The listing builds one solid part. Answer for the finished solid, in the listing's coordinates (mm). A direction names the side the tool comes from. Give positions to 0.01 mm unless a question says otherwise; leave off trailing zeros. Write each loop counter-clockwise with the first axis right and the second up, starting at its lowest first coordinate (ties: lowest second). Pieces come first, ordered by that corner, then holes. Notation, with made-up numbers: M 49,20 L 100,20 A21 ccw 100,55 Z; hole C -10,88.5 d3. An arc over 180 degrees is marked long. Return JSON: item names as keys, results as strings.
Autodesk Inventor part; units mm, degrees
ref_plane "YZ Plane" through (0, 0, 0) normal (1, 0, 0) x (0, 1, 0)
ref_plane "XZ Plane" through (0, 0, 0) normal (0, 1, 0) x (-1, 0, 0)
ref_plane "XY Plane" through (0, 0, 0) normal (0, 0, 1) x (1, 0, 0)
ref_plane "작업 평면1" through (0, 0, 0) normal (0, 0, 1) x (1, 0, 0)
sketch "스케치1" plane through (0, 0, 0) normal (0, 0, 1) x (1, 0, 0)
  circle A0 centre (-7.7782, -7.7782) radius 1.55
  circle A1 centre (7.7782, -7.7782) radius 1.55
  circle A2 centre (7.7782, 7.7782) radius 1.55
  circle A3 centre (-7.7782, 7.7782) radius 1.55
  circle A4 centre (0, 0) radius 5
  circle A5 centre (0, 0) radius 13.9
  circle A6 centre (0, 11) radius 1.55
  circle A7 centre (11, 0) radius 1.55
  circle A8 centre (0, -11) radius 1.55
  circle A9 centre (-11, 0) radius 1.55
  line L0 (13.9, 0) -> (13.9, 13.9)
  line L1 (13.9, 13.9) -> (-13.9, 13.9)
  line L2 (-13.9, 13.9) -> (13.9, 13.9)
  line L3 (13.9, 28.9) -> (-13.9, 28.9)
  line L4 (3.1, 28.9) -> (-3.1, 28.9)
  circle A10 centre (0, 0) radius 5.1
  circle A11 centre (-7.7782, 7.7782) radius 1.35
  circle A12 centre (-11, 0) radius 1.35
  circle A13 centre (-7.7782, -7.7782) radius 1.35
  circle A14 centre (0, -11) radius 1.35
  circle A15 centre (7.7782, -7.7782) radius 1.35
  circle A16 centre (11, 0) radius 1.35
  circle A17 centre (7.7782, 7.7782) radius 1.35
  circle A18 centre (0, 11) radius 1.35
  circle A19 centre (0, 0) radius 13.9
  line L5 (-5.1, 0) -> (-5.1, -12.9306)
  line L6 (5.1, 0) -> (5.1, -12.9306)
  line L7 (6.05, 28.9) -> (-6.05, 28.9)
  line L8 (-6.05, 28.9) -> (-6.05, 22.8)
  line L9 (-6.05, 22.8) -> (6.05, 22.8)
  line L10 (6.05, 22.8) -> (6.05, 28.9)
  line L11 (13.9, 28.9) -> (20.9, 28.9)
  line L12 (20.9, 28.9) -> (20.9, 13.9)
  line L13 (20.9, 13.9) -> (13.9, 13.9)
  line L14 (-13.9, 28.9) -> (-20.9, 28.9)
  line L15 (-20.9, 28.9) -> (-20.9, 13.9)
  line L16 (-20.9, 13.9) -> (-13.9, 13.9)
  line L17 (-20.9, 13.9) -> (-13.9, 0)
  line L18 (13.9, 0) -> (20.9, 13.9)
  circle A20 centre (-10.9, 25.9) radius 1.35
  circle A21 centre (10.9, 25.9) radius 1.35
  point P0 (0, 0)
  point P1 (0, 13.9)
  dimension "d24" = 0.1
  dimension "d25" = 2.7
  dimension "d28" = 360
  dimension "d30" = 12.1
  dimension "d31" = 6.1
  dimension "d39" = 2.7
  dimension "d40" = 2.7
extrude "돌출7" add sketch "스케치1" along normal blind 6 contours A0 | A1 | A2 | A3 | A5 L6 A10 L5 | L17 L16 L1 A5 | L1 L0 A5 | L1 L16 L15 L14 L3 L8 L9 L10 L11 L12 L13 | L0 L13 L18 | A6 | A7 | A9 picked at (-7.5104, -2.4224)
fillet "모깎기3" radius 1 2 edges at (-5.1, -12.9306, 3) (5.1, -12.9306, 3)
sketch "스케치2" plane through (0, 0, 6) normal (0, 0, 1) x (1, 0, 0)
  line L0 (-6.05, 22.8) -> (-6.05, 28.9)
  line L1 (6.05, 22.8) -> (-6.05, 22.8)
  line L2 (6.05, 28.9) -> (6.05, 22.8)
  circle A0 centre (-6.05, 22.8) radius 1
  circle A1 centre (6.05, 22.8) radius 1
  point P0 (0, 0)
  dimension "d47" = 2
  dimension "d48" = 2
extrude "돌출8" cut sketch "스케치2" against normal blind 10
properties part number "leg_between_64" material "PMMA 플라스틱"
Item 1: Find the intervals of material crossed by line 1 (Y direction, x = -8, z = 1.9); line 2 (Y direction, x = -11, z = 3.55); line 3 (X direction, y = 27, z = 5.75), in increasing order.
Geometry results:
{"line 1": "y = -11.37 to -9.11, -6.45 to 6.45, 9.11 to 28.9", "line 2": "y = -8.5 to -1.35, 1.35 to 24.55, 27.25 to 28.9", "line 3": "x = -20.9 to -11.68, -10.12 to -6.05, 6.05 to 10.12, 11.68 to 20.9"}
Item 2: A cutting plane is placed at C-C, the plane z = 4.9. Count the separate pieces of the cut face and the enclosed holes in it, plus the area to 3 significant figures.
Geometry results:
{"separate pieces": "1", "enclosed holes": "9", "area": "1,100 mm2"}
Item 3: A cutting plane is placed at B-B, the plane x = 0. Write down the section's boundary in (y, z), plus the area to 3 significant figures.
Geometry results:
{"outline": "M 5.1,0 L 9.65,0 L 9.65,6 L 5.1,6 Z; M 12.35,0 L 22.8,0 L 22.8,6 L 12.35,6 Z", "area": "90.0 mm2"}
Item 4: A cutting plane is placed at A-A, the plane y = 25.9. Write down the section's boundary in (x, z), plus the area to 3 significant figures.
Geometry results:
{"outline": "M -20.9,0 L -12.25,0 L -12.25,6 L -20.9,6 Z; M -9.55,0 L -6.05,0 L -6.05,6 L -9.55,6 Z; M 6.05,0 L 9.55,0 L 9.55,6 L 6.05,6 Z; M 12.25,0 L 20.9,0 L 20.9,6 L 12.25,6 Z", "area": "146 mm2"}
Item 5: Which of the six approach directions +Z, -Z, +X, -X, +Y, -Y give full straight-line access (tool end or side, diameter ignored) to faces 4 (the flat face through (5.1, -6, 3)), 5 (the cylindrical face through (12.247, 0.517, 2.958))?
Geometry results:
{"face 4": "+Z, -Z, -Y", "face 5": "+Z, -Z"}
Item 6: Given pin 1 Ø3 at (x, y) = (-7.78, 7.78) entering from +Z; pin 2 Ø1.5 at (y, z) = (-2, 4.5) entering from -X, each flat-ended and moving along its own axis, determine where each tip first touches the part or whether it passes through.
Geometry results:
{"pin 1": "stops at z = 6", "pin 2": "stops at x = -13.84"}
Item 7: Determine the mould class of faces 1 (the flat face through (20.9, 22, 3)), 2 (the cylindrical face through (6.78, 6.87, 2.96)), 3 (the flat face through (-20.9, 22, 3)) for opening direction X: +X half, -X half, draft (parallel to the pull), parting line (faces both ways), or undercut.
Geometry results:
{"face 1": "+X half", "face 2": "undercut", "face 3": "-X half"}
Item 8: A cutting plane is placed at D-D, the plane y = -3.5. Write down the section's boundary in (x, z).
Geometry results:
{"outline": "M -13.45,0 L -5.1,0 L -5.1,6 L -13.45,6 Z; M 5.1,0 L 13.45,0 L 13.45,6 L 5.1,6 Z"}
